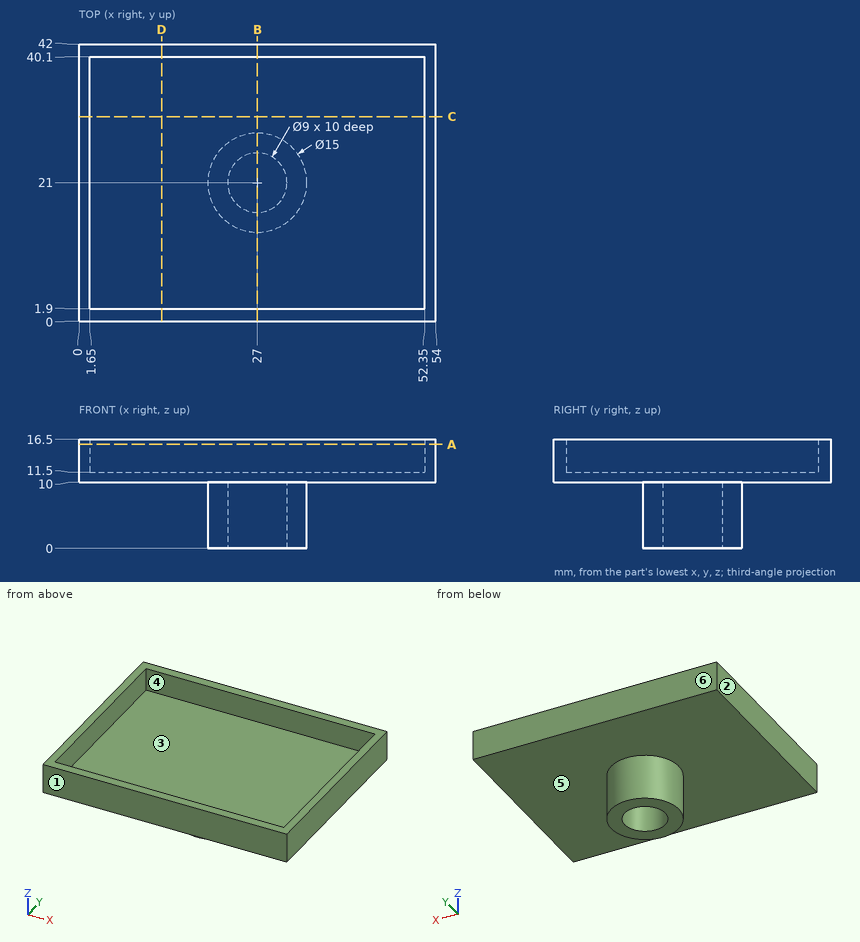
Geometry check sheet. Reference: drawing and pictorial views, mm from the part's lowest x, y, z. A direction names the side the tool comes from. Give positions to 0.01 mm unless a question says otherwise; leave off trailing zeros. Order: outer loops, then holes, each group sorted by start corner. A loop starts at its lowest first (then second) coordinate and runs counter-clockwise, first axis right, second up. Notation, with made-up numbers: M 8.5,-12 L 13.5,-12 A22 cw 13.5,12 Z; hole C -2,28 d10. An arc over 180 degrees is marked long. Answer in a Markdown table with one row per item. Add a question column.
Item 1: Scan lines: probe 1 along Y at (x, z) = (27, 3.5); probe 2 along Y at (x, z) = (17, 12.5); probe 3 along X at (y, z) = (14.5, 15.5). Record each from-to range of solid material in increasing order. Write a range as from..to.
Item 2: Section check A-A, the plane z = 15.75. Enter the section's corners in (x, y).
Item 3: Gauge pin test, flat ends, axial feed: pin 1 (4 mm diameter, centred on x = 24.5, y = 32, fed in from -Z); pin 2 (8 mm diameter, centred on y = 35, z = 7.5, fed in from +X); pin 3 (5.5 mm diameter, centred on x = 27, y = 21, fed in from +Z). Record the tip position at first contact, or that the pin passes through.
Item 4: Section check B-B, the plane x = 27. Enter the section's corners in (y, z).
Item 5: Section check C-C, the plane y = 31. Enter the section's corners in (x, z), and give its area (3 significant figures).
Item 6: Tool access check on the marked faces 4, 5 and 6. Record the directions out of +Z, -Z, +X, -X, +Y, -Y that give a thin tool (end or side, any length) a straight path to the whole face; none if there is none.
Item 7: Mould release check, pull along X, two halves, no side actions. Record for the marked faces 1, 2 and 3: released by +X, released by -X, zero draft, split by the parting line, or undercut.
Item 8: Section check D-D, the plane x = 12.5. Enter the section's corners in (y, z).
Filled sheet:
| question | item | result |
|---|---|---|
| 1 | probe 1 | y = 13.5..16.5, 25.5..28.5 |
| 1 | probe 2 | y = 0..1.9, 40.1..42 |
| 1 | probe 3 | x = 0..1.65, 52.35..54 |
| 2 | outline | M 0,0 L 54,0 L 54,42 L 0,42 Z; hole M 1.65,1.9 L 52.35,1.9 L 52.35,40.1 L 1.65,40.1 Z |
| 3 | pin 1 | stops at z = 10 |
| 3 | pin 2 | stops at x = 54 |
| 3 | pin 3 | stops at z = 11.5 |
| 4 | outline | M 0,10 L 13.5,10 L 13.5,0 L 16.5,0 L 16.5,10 L 25.5,10 L 25.5,0 L 28.5,0 L 28.5,10 L 42,10 L 42,16.5 L 40.1,16.5 L 40.1,11.5 L 1.9,11.5 L 1.9,16.5 L 0,16.5 Z |
| 5 | outline | M 0,10 L 54,10 L 54,16.5 L 52.35,16.5 L 52.35,11.5 L 1.65,11.5 L 1.65,16.5 L 0,16.5 Z |
| 5 | area | 97.5 mm^2 |
| 6 | face 4 | +Z |
| 6 | face 5 | -Z |
| 6 | face 6 | +Z, -Z, +X, -X, +Y |
| 7 | face 1 | zero draft |
| 7 | face 2 | released by -X |
| 7 | face 3 | undercut |
| 8 | outline | M 0,10 L 42,10 L 42,16.5 L 40.1,16.5 L 40.1,11.5 L 1.9,11.5 L 1.9,16.5 L 0,16.5 Z |
